Design review of the part built by this model. Coordinates are the model's own, in mm. Coordinates: 2 decimals unless noted, no trailing zeros. Order: outer loops, then holes, each group sorted by start corner. A loop starts at its lowest first (then second) coordinate and runs counter-clockwise, first axis right, second up. Notation, with made-up numbers: M 8.5,70 L 18.5,70 A36 cw 18.5,108 Z; hole C -20,-11 d11. An arc over 180 degrees is marked long. Answer in a Markdown table with one row per item.
from build123d import *
from build123d.topology import SkipClean

# Parameters (mm, degrees)
SKETCH1_R           = 12
BOSS_EXTRUDE1_DEPTH = 3.175
BOSS_EXTRUDE2_START = 3.81
SKETCH2_R           = 12
BOSS_EXTRUDE2_DEPTH = 3.81
SKETCH3_R           = 3.937
CUT_EXTRUDE1_DEPTH  = 134.099089527
SKETCH4_R           = 1.27
CUT_EXTRUDE2_DEPTH  = 134.099089527


with BuildPart() as part:
    # Sketch1 → Boss-Extrude1 (new body)
    with BuildSketch(Plane.XY):
        with BuildLine():
            ThreePointArc((79.156979953, 34.616777747), (78.764409425, 33.207913627), (78.648230314, 31.75))
            Line((78.648230314, 31.75), (93.886132052, 31.75))
            ThreePointArc((93.886132052, 31.75), (93.886918896, 31.813218964), (93.887181183, 31.876442281))
            ThreePointArc((93.887181183, 31.876442281), (87.66085737, 39.367908538), (79.156979953, 34.616777747))
        make_face()
        with BuildLine():
            ThreePointArc((87.4395, 24.347161532), (88.598049964, 24.621688616), (89.699693339, 25.073335615))
            ThreePointArc((89.699693339, 25.073335615), (92.723044454, 27.828451492), (93.886132052, 31.75))
            Line((93.886132052, 31.75), (78.648230314, 31.75))
            ThreePointArc((78.648230314, 31.75), (79.141141445, 29.177561465), (80.476005529, 26.924))
            Line((80.476005529, 26.924), (87.4395, 26.924))
            Line((87.4395, 26.924), (87.4395, 24.347161532))
        make_face()
        with BuildLine():
            Line((87.4395, 26.924), (80.476005529, 26.924))
            ThreePointArc((80.476005529, 26.924), (82.246043304, 25.403819152), (84.393093646, 24.490496444))
            ThreePointArc((84.393093646, 24.490496444), (85.909052633, 24.264862685), (87.4395, 24.347161532))
            Line((87.4395, 24.347161532), (87.4395, 26.924))
        make_face()
        with BuildLine():
            ThreePointArc((89.699693339, 25.073335615), (94.483227873, 27.711788353), (99.06, 30.694537484))
            Line((99.06, 30.694537484), (99.06, 31.75))
            Line((99.06, 31.75), (93.886132052, 31.75))
            ThreePointArc((93.886132052, 31.75), (92.723044454, 27.828451492), (89.699693339, 25.073335615))
        make_face()
        with BuildLine():
            ThreePointArc((99.06, 30.694537484), (106.888760949, 37.054762789), (113.784062988, 44.416608597))
            ThreePointArc((113.784062988, 44.416608597), (96.436063978, 43.110085278), (96.014300162, 60.502100346))
            ThreePointArc((96.014300162, 60.502100346), (86.225733854, 48.445051897), (79.156979953, 34.616777747))
            ThreePointArc((79.156979953, 34.616777747), (87.66085737, 39.367908538), (93.887181183, 31.876442281))
            ThreePointArc((93.887181183, 31.876442281), (93.886918896, 31.813218964), (93.886132052, 31.75))
            Line((93.886132052, 31.75), (99.06, 31.75))
            Line((99.06, 31.75), (99.06, 30.694537484))
        make_face()
        with Locations((104.48925, 52.0065)):
            Circle(SKETCH1_R)
    extrude(amount=BOSS_EXTRUDE1_DEPTH)

    # Sketch2 → Boss-Extrude2 (add)
    with SkipClean():  # the faces are left unmerged after this step: merging them gives an invalid solid
        with BuildSketch(Plane(origin=(0, 0, 0), x_dir=(-1, 0, 0), z_dir=(0, 0, -1)).offset(BOSS_EXTRUDE2_START)):
            with Locations((-104.48925, 52.0065)):
                Circle(SKETCH2_R)
        extrude(amount=-BOSS_EXTRUDE2_DEPTH)

    # Sketch3 → Cut-Extrude1 (cut, through all)
    with SkipClean():  # the faces are left unmerged after this step: merging them gives an invalid solid
        with BuildSketch(Plane(origin=(0, 0, -3.81), x_dir=(-1, 0, 0), z_dir=(0, 0, -1))):
            with Locations((-104.48925, 52.0065)):
                Circle(SKETCH3_R)
        extrude(amount=-CUT_EXTRUDE1_DEPTH, mode=Mode.SUBTRACT)

    # Sketch4 → Cut-Extrude2 (cut, through all)
    with SkipClean():  # the faces are left unmerged after this step: merging them gives an invalid solid
        with BuildSketch(Plane(origin=(0, 0, -3.81), x_dir=(-1, 0, 0), z_dir=(0, 0, -1))):
            with Locations((-112.99825, 52.0065)):
                Circle(SKETCH4_R)
            with Locations((-95.98025, 52.0065)):
                Circle(SKETCH4_R)
            with Locations((-104.48925, 60.5155)):
                Circle(SKETCH4_R)
            with Locations((-104.48925, 43.4975)):
                Circle(SKETCH4_R)
        extrude(amount=-CUT_EXTRUDE2_DEPTH, mode=Mode.SUBTRACT)


solid = part.part
(1) Add section C-C, the plane z = 1. Give the boundary of the cut face in (x, y).
Return value:
| item | result |
|---|---|
| outline | M 79.16,34.62 A7.62 ccw 89.7,25.07 A74.31 ccw 113.78,44.42 A12 ccw 96.01,60.5 A74.31 ccw Z; hole C 95.98,52.01 d2.54; hole C 104.49,52.01 d7.87; hole C 104.49,43.5 d2.54; hole C 104.49,60.52 d2.54; hole C 113,52.01 d2.54 |
(2) Insertion check: pin 1 Ø2 at (y, z) = (39.5, 1) entering from -X; pin 2 Ø10.5 at (x, y) = (96, 36.5) entering from -Z; pin 3 Ø2 at (x, z) = (86.5, 1) entering from +Y. Each pin has a flat end and moves straight along its axis. Give the tip position at first contact, or say it passes through.
Return value:
| item | result |
|---|---|
| pin 1 | stops at x = 80.78 |
| pin 2 | stops at z = 0 |
| pin 3 | stops at y = 50.34 |
(3) For line 1 along Y through (x, z) = (105, -2); line 2 along Z through (x, y) = (91, 47.5) (3 decimals); line 3 along X through (y, z) = (50.5, -2.75), list the stretches that pass through material, from the lowest coordinate up. Write a range as from..to.
Return value:
| item | result |
|---|---|
| line 1 | y = 40.02..42.33, 44.66..48.1, 55.91..59.35, 61.68..64 |
| line 2 | z = 0..3.175 |
| line 3 | x = 92.58..100.85, 108.13..116.39 |
(4) Add section D-D, the plane y = 35.5. Give the boundary of the cut face in (x, z) (3 decimals).
Return value:
| item | result |
|---|---|
| outline | M 79.504,0 L 105.167,0 L 105.167,3.175 L 79.504,3.175 Z |
(5) Add section B-B, the plane x = 93.5. Give the boundary of the cut face in (y, z) (3 decimals).
Return value:
| item | result |
|---|---|
| outline | M 27.132,0 L 47.186,0 L 47.186,-3.81 L 56.827,-3.81 L 56.827,0 L 57.868,0 L 57.868,3.175 L 27.132,3.175 Z |
(6) Add section A-A, the plane y = 49. Give the boundary of the cut face in (x, z) (3 decimals).
Return value:
| item | result |
|---|---|
| outline | M 86.591,0 L 92.872,0 L 92.872,-3.81 L 101.947,-3.81 L 101.947,3.175 L 86.591,3.175 Z; M 107.031,-3.81 L 116.107,-3.81 L 116.107,3.175 L 107.031,3.175 Z |
(7) Draft analysis for pull direction Y (two halves, no side actions). For faces 1 (the cylindrical face through (86.345, 48.627, 1.565)), 2 (the cylindrical face through (114.267, 52.062, -0.366)), 3 (the flat face through (92, 39, 0)), state which applies: pulls with the +Y half, pulls with the -Y half, needs draft (parallel to the pull), parting line crosses it, or undercut.
Return value:
| item | result |
|---|---|
| face 1 | pulls with the +Y half |
| face 2 | undercut |
| face 3 | needs draft |
